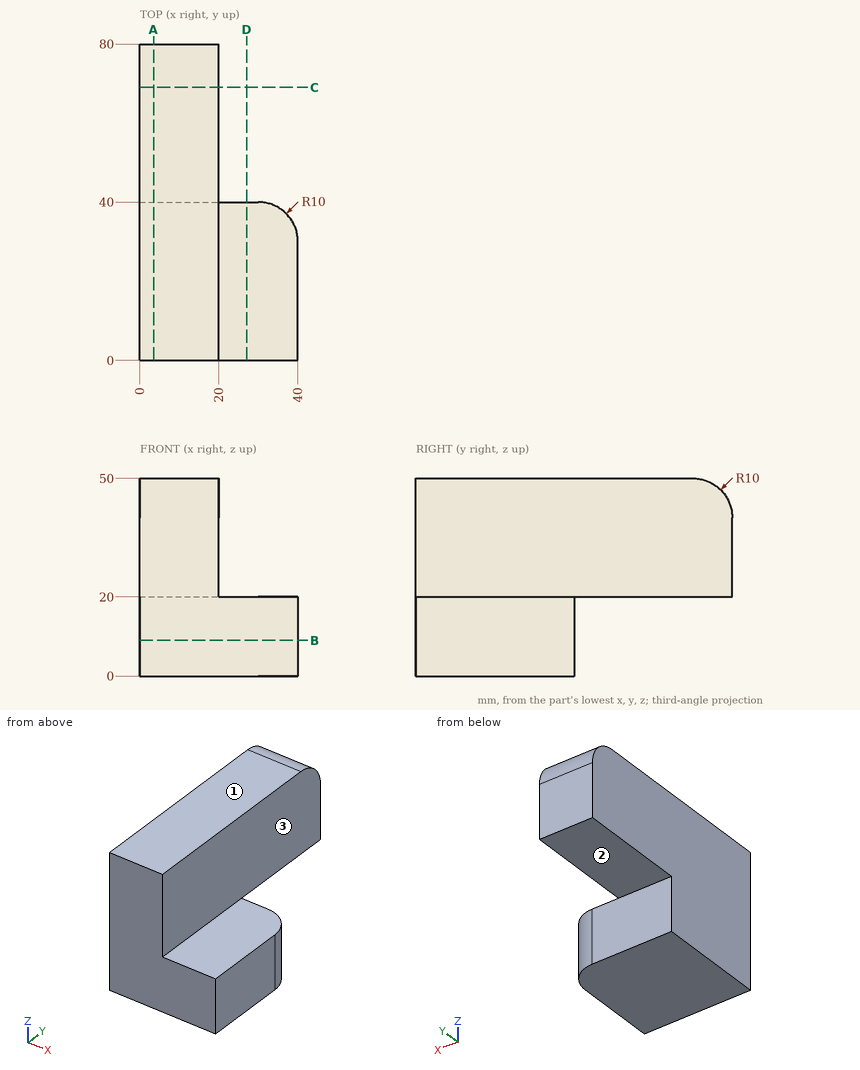
Study the drawing (mm; zero at the part's minimum x, y, z) and answer. A direction names the side the tool comes from. Round coordinates to 2 decimals unless told otherwise and drop trailing zeros. Write each loop counter-clockwise with the first axis right and the second up, starting at its lowest first coordinate (ties: lowest second). Pieces come first, ordered by that corner, then holes.
1) A cutting plane is placed at D-D on x = 27. Determine the outline of the cut face in (y, z).
2) A cutting plane is placed at A-A on x = 3.5. Determine the outline of the cut face in (y, z).
3) Flat-ended cylindrical pins translate along their axes: P1, Ø16, axis at x = 9.5, y = 69.5, coming from the -Z side; P2, Ø6, axis at x = 28.5, y = 28, coming from the +Z side; P3, Ø10, axis at x = 8.5, z = 7, coming from the +Y side. Find the tip coordinate at first contact, or state that the pin passes through.
4) Consider probe 1 along X at (y, z) = (69, 33); probe 2 along Y at (x, z) = (18, 19.5). Determine where each line is inside the solid, lowest interval first.
5) A cutting plane is placed at B-B on z = 9. Determine the outline of the cut face in (x, y), and give its area (3 significant figures).
6) A cutting plane is placed at C-C on y = 69. Determine the outline of the cut face in (x, z).
7) Which of the six approach directions +Z, -Z, +X, -X, +Y, -Y give full straight-line access (tool end or side, diameter ignored) to the marked faces 1, 2 and 3?
Entries:
1. outline: (0, 0) - (40, 0) - (40, 20) - (0, 20) - close
2. outline: (0, 0) - (40, 0) - (40, 20) - (80, 20) - (80, 40) arc R10 ccw to (70, 50) - (0, 50) - close
3. P1: stops at z = 20
3. P2: stops at z = 20
3. P3: stops at y = 40
4. probe 1: x = 0 to 20
4. probe 2: y = 0 to 40
5. outline: (0, 0) - (40, 0) - (40, 30) arc R10 ccw to (30, 40) - (0, 40) - close
5. area: 1,580 mm2
6. outline: (0, 20) - (20, 20) - (20, 50) - (0, 50) - close
7. face 1: +Z, +X, -X, +Y, -Y
7. face 2: -Z, +X, -X, +Y
7. face 3: +Z, +X, +Y, -Y
